```python
from build123d import *

# Parameters (mm, degrees)
SKETCH1_W           = 26.67
SKETCH1_H           = 34.163
SKETCH1_R           = 1.143
BOSS_EXTRUDE1_DEPTH = 1.651
SKETCH2_W           = 16.51
SKETCH2_H           = 15.24
BOSS_EXTRUDE2_DEPTH = 4.826


with BuildPart() as part:
    # Sketch1 → Boss-Extrude1 (new body)
    with BuildSketch(Plane(origin=(0, 0, 0), x_dir=(1, 0, 0), z_dir=(0, 1, 0))):
        with Locations((10.16, -14.2875)):
            Rectangle(SKETCH1_W, SKETCH1_H)
        Circle(SKETCH1_R, mode=Mode.SUBTRACT)
        with Locations((20.32, 0)):
            Circle(SKETCH1_R, mode=Mode.SUBTRACT)
    extrude(amount=BOSS_EXTRUDE1_DEPTH)

    # Sketch2 → Boss-Extrude2 (add)
    with BuildSketch(Plane(origin=(0, 1.651, 0), x_dir=(1, 0, 0), z_dir=(0, 1, 0))):
        with Locations((9.271, -13.716)):
            Rectangle(SKETCH2_W, SKETCH2_H)
    extrude(amount=BOSS_EXTRUDE2_DEPTH)


solid = part.part
```
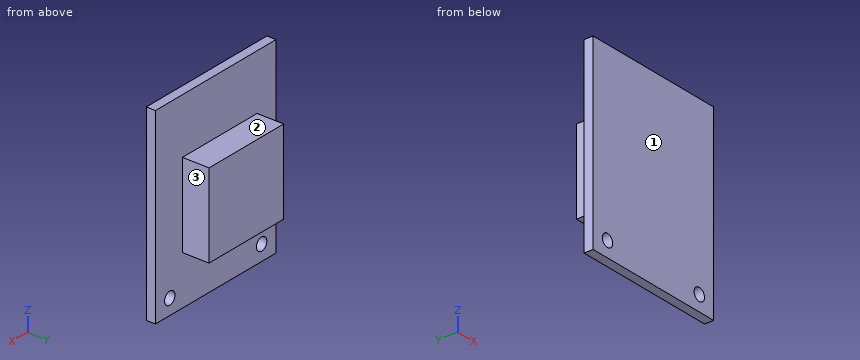
Could you check a few things on this model? Use its own coordinates, in mm. Face numbers are marked on the shaded views. A direction names the side the tool comes from. Round coordinates to 2 decimals unless told otherwise and drop trailing zeros. Loops run counter-clockwise (first coordinate to the right, second up) from the corner with the lowest first, then second, coordinate; pieces in that order, holes last. Notation, with made-up numbers: (-39.5, -13.75) -> (16.5, -13.75) arc R9 ccw to (16.5, 3.25) -> close; hole circle Ø6 at (25, 17.5). An arc over 180 degrees is marked (long way). Put each result on its own line as item: value.
Q1. I want a section at A-A on x = 20.32. Write out the boundary of the cut face in (y, z).
Checks:
outline: (0, -2.79) -> (1.65, -2.79) -> (1.65, -1.14) -> (0, -1.14) -> close; (0, 1.14) -> (1.65, 1.14) -> (1.65, 31.37) -> (0, 31.37) -> close
Q2. I want a section at B-B on x = 6.25. Write out the boundary of the cut face in (y, z), and give its area (3 significant figures).
Checks:
outline: (0, -2.79) -> (1.65, -2.79) -> (1.65, 6.1) -> (6.48, 6.1) -> (6.48, 21.34) -> (1.65, 21.34) -> (1.65, 31.37) -> (0, 31.37) -> close
area: 130 mm2
Q3. Which directions (+Z, -Z, +X, -X, +Y, -Y) give clear straight access to the entire face, cutting with the end or side of a thin tool? Please do the marked faces 1, 2 and 3.
Checks:
face 1: +Z, -Z, +X, -X, -Y
face 2: +Z, +X, -X, +Y
face 3: +Z, -Z, +X, +Y
Q4. I want a section at C-C on z = 11. Write out the boundary of the cut face in (x, y) (3 decimals).
Checks:
outline: (-3.175, 0) -> (23.495, 0) -> (23.495, 1.651) -> (17.526, 1.651) -> (17.526, 6.477) -> (1.016, 6.477) -> (1.016, 1.651) -> (-3.175, 1.651) -> close
Q5. I want a section at D-D on y = 3.25. Write out the boundary of the cut face in (x, z), and give its area (3 significant figures).
Checks:
outline: (1.02, 6.1) -> (17.53, 6.1) -> (17.53, 21.34) -> (1.02, 21.34) -> close
area: 252 mm2
Q6. For pin 1 Ø2 at (x, y) = (20.5, 4) entering from +Z; pin 2 Ø2.5 at (y, z) = (4, 15) entering from +X; pin 3 Ø3 at (x, y) = (0, 4.5) entering from +Z; pin 4 Ø3 at (x, z) = (10, 27.5) entering from +Y, each with a flat end and sliding along its axis, tell me the tip position at first contact or that it passes through.
Checks:
pin 1: through
pin 2: x = 17.53
pin 3: z = 21.34
pin 4: y = 1.65
Q7. Please list where these lines run through material, in increasing order: line 1 (X direction, y = 0.75, z = 0) (3 decimals); line 2 (Z direction, x = 0, y = 1); line 3 (Y direction, x = 12.5, z = -1). Write a range as from..to.
Checks:
line 1: -3.175..-1.143, 1.143..19.177, 21.463..23.495
line 2: -2.79..-1.14, 1.14..31.37
line 3: 0..1.65
